Read the model definition and answer for the solid it produces. Units are mm, in the model's axes. Face numbers are marked on the shaded views. A direction names the side the tool comes from. Give positions to 0.01 mm unless a question says otherwise; leave off trailing zeros. Write each loop counter-clockwise with the first axis right and the second up, starting at its lowest first coordinate (ties: lowest second). Pieces come first, ordered by that corner, then holes. Notation, with made-up numbers: M 37.25,-5.75 L 54.25,-5.75 A28 ccw 54.25,20.25 Z; hole C 49,-7.75 d9. An arc over 180 degrees is marked long. Use a Markdown table: item, result. Add a question column.
Item 1: For the marked faces 1 and 2, determine the directions among +Z, -Z, +X, -X, +Y, -Y from which every point of the face is accessible in a straight line to the end or side of a thin tool.
Item 2: A cutting plane is placed at A-A on y = 0. Determine the outline of the cut face in (x, z).
Item 3: A cutting plane is placed at B-B on z = 9.5. Determine the outline of the cut face in (x, y), then the cut area to 3 significant figures.
Item 4: Given P1, Ø6, axis at x = 2.5, z = 20.5, coming from the +Y side; P2, Ø2, axis at x = -3.5, z = 21.5, coming from the +Y side, each flat-ended and moving along its own axis, determine where each tip first touches the part or whether it passes through.
Item 5: Consider probe 1 along Z at (x, y) = (-2.75, -4.25); probe 2 along X at (y, z) = (-2.25, 21.75); probe 3 along X at (y, z) = (-2, 10.5). Determine where each line is inside the solid, lowest interval first. Write a range as [from, to].
from build123d import *

# Parameters (mm, degrees)
ESQUISSE1_W        = 4
ESQUISSE1_H        = 25
CHANFREIN1_SIZE    = 0.8
BOSS_EXTRU_1_DEPTH = 4.5


with BuildPart() as part:
    # Esquisse1 → Base-Révolution (revolve)
    with BuildSketch(Plane(origin=(0, 0, 0), x_dir=(1, 0, 0), z_dir=(0, 1, 0))):
        with Locations((2, -12.5)):
            Rectangle(ESQUISSE1_W, ESQUISSE1_H)
    revolve(axis=Axis((0, 0, 0), (0, 0, 1)))

    # Chanfrein1
    chanfrein1_edges = [part.edges().sort_by_distance(p)[0] for p in [
        (-4, 0, 25),
    ]]
    chamfer(chanfrein1_edges, length=CHANFREIN1_SIZE)

    # Esquisse6 → Boss.-Extru.1 (add)
    with BuildSketch(Plane.XY):
        Polygon((6.5, -3.75277675), (6.5, 3.75277675), (0, 7.505553499), (-6.5, 3.75277675), (-6.5, -3.75277675), (0, -7.505553499), align=None)
    extrude(amount=-BOSS_EXTRU_1_DEPTH)

    # Esquisse7 → Enlèvement de matière-Révolution1 (revolve, cut)
    with BuildSketch(Plane(origin=(0, 0, 0), x_dir=(1, 0, 0), z_dir=(0, 1, 0))):
        Polygon((-5.5, 4.5), (-13.294228634, 4.5), (-13.294228634, 0), align=None)
    revolve(axis=Axis((0, 0, -6.239446496), (0, 0, 1)), mode=Mode.SUBTRACT)


solid = part.part
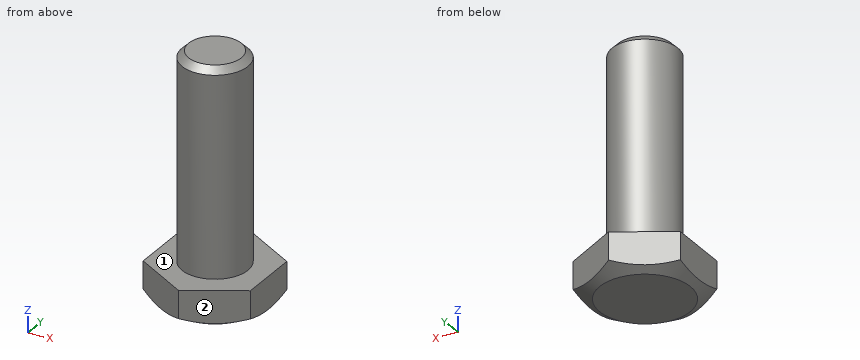
Filled in:
| question | item | result |
|---|---|---|
| 1 | face 1 | +Z |
| 1 | face 2 | +Z, -Z, +X, -Y |
| 2 | outline | M -6.5,-3.92 L -5.5,-4.5 L 5.5,-4.5 L 6.5,-3.92 L 6.5,0 L 4,0 L 4,24.2 L 3.2,25 L -3.2,25 L -4,24.2 L -4,0 L -6.5,0 Z |
| 3 | outline | C 0,0 d8 |
| 3 | area | 50.3 mm² |
| 4 | P1 | y = 4 |
| 4 | P2 | y = 3.12 |
| 5 | probe 1 | [-4.5, 0] |
| 5 | probe 2 | [-3.31, 3.31] |
| 5 | probe 3 | [-3.46, 3.46] |
